Design review of the part built by this model. Coordinates are the model's own, in mm. Face numbers are marked on the shaded views. A direction names the side the tool comes from. Give positions to 0.01 mm unless a question says otherwise; leave off trailing zeros. Order: outer loops, then holes, each group sorted by start corner. A loop starts at its lowest first (then second) coordinate and runs counter-clockwise, first axis right, second up. Notation, with made-up numbers: (2, -9) -> (14, -9) arc R22 cw to (14, 21) -> close; hole circle Ø5 at (-31, 75.5). An arc over 180 degrees is marked (long way). One line per item, written item: value.
Autodesk Inventor part; units mm, degrees
ref_plane "YZ Plane" through (0, 0, 0) normal (1, 0, 0) x (0, 1, 0)
ref_plane "XZ Plane" through (0, 0, 0) normal (0, 1, 0) x (-1, 0, 0)
ref_plane "XY Plane" through (0, 0, 0) normal (0, 0, 1) x (1, 0, 0)
sketch "Sketch1" plane through (0, 0, 0) normal (0, 1, 0) x (-1, 0, 0)
  line L0 (0, 0) -> (25.4, 0)
  line L1 (25.4, 0) -> (25.4, -25.4)
  line L2 (25.4, -25.4) -> (0, -25.4)
  line L3 (0, -25.4) -> (0, 0)
  line L4 (23.4, -23.4) -> (23.4, -2)
  line L5 (23.4, -2) -> (2, -2)
  line L6 (2, -2) -> (2, -23.4)
  line L7 (2, -23.4) -> (23.4, -23.4)
  dimension "d0" = 25.4
  dimension "d1" = 25.4
  dimension "d2" = 2
extrude "Extrusion1" add sketch "Sketch1" along normal blind 152.4
sketch "Sketch2" plane through (-25.4, 0, 0) normal (0, 0, 1) x (1, 0, 0)
  line L0 (25.4, 0) -> (0, 0)
  circle A0 centre (12.7, 5.4) radius 2
  dimension "d6" = 4
extrude "Extrusion2" cut sketch "Sketch2" against normal through all
sketch "Sketch3" plane through (0, 0, 0) normal (1, 0, 0) x (0, 0, -1)
  line L0 (0, 0) -> (25.4, 0)
  circle A0 centre (12.7, 15.4) radius 2
  dimension "d10" = 4
extrude "Extrusion3" cut sketch "Sketch3" against normal through all
sketch "Sketch4" plane through (0, 0, 0) normal (1, 0, 0) x (0, 0, -1)
  line L0 (23.4, 0) -> (2, 0)
  line L1 (12.7, 35.4) -> (22.7, 35.4)
  line L2 (22.7, 35.4) -> (22.7, 62.4)
  line L3 (23.4, 0) -> (23.4, 152.4)
  line L4 (22.7, 62.4) -> (2.7, 62.4)
  line L5 (2.7, 62.4) -> (2.7, 35.4)
  line L6 (2.7, 35.4) -> (12.7, 35.4)
  point P0 (0, 0)
  dimension "d15" = 10
  dimension "d16" = 20
extrude "Extrusion4" cut sketch "Sketch4" against normal blind 10
properties part number "Metal_Bone"
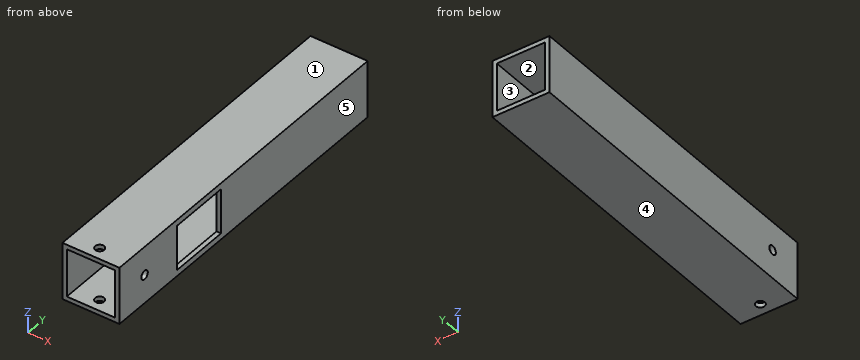
Item 1: Add section C-C on x = -12.7. Give the boundary of the cut face in (y, z), plus the area to 3 significant figures.
Returned:
outline: (0, -25.4) -> (3.4, -25.4) -> (3.4, -23.4) -> (0, -23.4) -> close; (0, -2) -> (3.4, -2) -> (3.4, 0) -> (0, 0) -> close; (7.4, -25.4) -> (152.4, -25.4) -> (152.4, -23.4) -> (7.4, -23.4) -> close; (7.4, -2) -> (152.4, -2) -> (152.4, 0) -> (7.4, 0) -> close
area: 594 mm²
Item 2: Clearance check with a flat-ended pin moving along its axis: P1, Ø2.5, axis at y = 15.4, z = -12.7, coming from the -X side. State where the tip first meets the part, or that it passes through.
Returned:
P1: through
Item 3: Draft analysis for pull direction X (two halves, no side actions). For the marked faces 3, 4 and 5, state which applies: pulls with the +X half, pulls with the -X half, needs draft (parallel to the pull), parting line crosses it, or undercut.
Returned:
face 3: undercut
face 4: needs draft
face 5: pulls with the +X half
Item 4: Add section B-B on y = 15.4. Give the boundary of the cut face in (x, z).
Returned:
outline: (-25.4, -25.4) -> (0, -25.4) -> (0, -14.7) -> (-2, -14.7) -> (-2, -23.4) -> (-23.4, -23.4) -> (-23.4, -14.7) -> (-25.4, -14.7) -> close; (-25.4, -10.7) -> (-23.4, -10.7) -> (-23.4, -2) -> (-2, -2) -> (-2, -10.7) -> (0, -10.7) -> (0, 0) -> (-25.4, 0) -> close
Item 5: Add section A-A on z = -12.7. Give the boundary of the cut face in (x, y).
Returned:
outline: (-25.4, 0) -> (-23.4, 0) -> (-23.4, 13.4) -> (-25.4, 13.4) -> close; (-25.4, 17.4) -> (-23.4, 17.4) -> (-23.4, 152.4) -> (-25.4, 152.4) -> close; (-2, 0) -> (0, 0) -> (0, 13.4) -> (-2, 13.4) -> close; (-2, 17.4) -> (0, 17.4) -> (0, 35.4) -> (-2, 35.4) -> close; (-2, 62.4) -> (0, 62.4) -> (0, 152.4) -> (-2, 152.4) -> close
Item 6: To check wall thickness, follow line 1 along Y through (x, z) = (-0.8, -12.7); line 2 along Y through (x, z) = (-12.7, -0.85); line 3 along Z through (x, y) = (-22.75, 54). State the ranges of each line that lie inside material, in increasing order. Write a range as from..to.
Returned:
line 1: 0..13.4, 17.4..35.4, 62.4..152.4
line 2: 0..3.4, 7.4..152.4
line 3: -25.4..-23.4, -2..0
Item 7: Machinability: for the marked faces 1 and 2, which of the approach directions +Z, -Z, +X, -X, +Y, -Y give a long, thin tool a straight path to every point of the face, cutting with its end or side? Answer none if there is none.
Returned:
face 1: +Z, +X, -X, +Y, -Y
face 2: +Y, -Y
Item 8: Add section D-D on y = 114. Give the boundary of the cut face in (x, z), plus the area to 3 significant figures.
Returned:
outline: (-25.4, -25.4) -> (0, -25.4) -> (0, 0) -> (-25.4, 0) -> close; hole (-23.4, -23.4) -> (-2, -23.4) -> (-2, -2) -> (-23.4, -2) -> close
area: 187 mm²
